Autodesk Inventor part; units mm, degrees
ref_plane "YZ Plane" through (0, 0, 0) normal (1, 0, 0) x (0, 1, 0)
ref_plane "XZ Plane" through (0, 0, 0) normal (0, 1, 0) x (-1, 0, 0)
ref_plane "XY Plane" through (0, 0, 0) normal (0, 0, 1) x (1, 0, 0)
sketch "Sketch1" plane through (0, 0, 0) normal (0, 0, 1) x (1, 0, 0)
  line L0 (232, 157.1) -> (-18, 157.1)
  line L1 (-18, 157.1) -> (-18, -92.9)
  line L2 (-18, -92.9) -> (232, -92.9)
  line L3 (232, -92.9) -> (232, 157.1)
  line L4 (-18, -42.8) -> (0, -42.8)
  line L5 (0, -42.8) -> (0, -92.9)
  line L6 (0, -92.9) -> (-18, -92.9)
  line L7 (-18, -92.9) -> (-18, -42.8)
  line L8 (0, 107) -> (0, 64.2)
  line L9 (0, 64.2) -> (-18, 64.2)
  line L10 (-18, 64.2) -> (-18, 107)
  line L11 (76.5522, 157.3937) -> (94.5522, 157.3937)
  line L12 (-18, -42.8) -> (-18, 0)
  line L13 (-18, 0) -> (0, 0)
  line L14 (0, 0) -> (0, -42.8)
  line L15 (0, -42.8) -> (-18, -42.8)
  line L16 (-18, -42.8) -> (0, -42.8)
  line L17 (0, -42.8) -> (0, 0)
  line L18 (0, 0) -> (-18, 0)
  line L19 (-18, 0) -> (-18, -42.8)
  line L20 (0, 0) -> (-18, 0)
  line L21 (-18, 0) -> (-18, 64.2)
  line L22 (-18, 64.2) -> (0, 64.2)
  line L23 (0, 64.2) -> (0, 0)
  line L24 (-18, 64.2) -> (-18, 107)
  line L25 (0, 64.2) -> (-18, 64.2)
  line L26 (-18, 64.2) -> (-18, 107)
  line L27 (76.5522, 157.3937) -> (94.5522, 157.3937)
  line L28 (0, 107) -> (0, 64.2)
  line L29 (76.5522, 157.3937) -> (94.5522, 157.3937)
  line L30 (0, 107) -> (0, 157.1)
  line L31 (0, 157.1) -> (-18, 157.1)
  line L32 (-18, 157.1) -> (-18, 107)
  line L33 (0, 64.2) -> (0, 107)
  line L34 (0, 107) -> (-18, 107)
  line L35 (232, -92.9) -> (94.5522, -92.9)
  line L36 (-18, -92.9) -> (107, -92.9)
  line L37 (107, -92.9) -> (107, 52.5886)
  line L38 (232, 157.1) -> (232, -92.9)
  line L39 (232, -42.8) -> (214, -42.8)
  line L40 (232, -92.9) -> (232, -42.8)
  line L41 (214, -42.8) -> (214, -92.9)
  line L42 (214, 107) -> (214, 64.2)
  line L43 (214, 107) -> (214, 64.2)
  line L44 (232, 64.2) -> (232, 107)
  line L45 (232, 64.2) -> (232, 107)
  line L46 (232, 64.2) -> (232, 107)
  line L47 (214, 107) -> (214, 157.1)
  line L48 (232, 157.1) -> (232, 107)
  line L49 (214, -42.8) -> (232, -42.8)
  line L50 (232, -42.8) -> (214, -42.8)
  line L51 (214, -42.8) -> (214, 0)
  line L52 (232, -42.8) -> (232, 0)
  line L53 (232, 0) -> (214, 0)
  line L54 (232, 0) -> (232, -42.8)
  line L55 (214, 0) -> (232, 0)
  line L56 (214, 0) -> (232, 0)
  line L57 (214, 64.2) -> (214, 0)
  line L58 (214, 64.2) -> (232, 64.2)
  line L59 (232, 0) -> (232, 64.2)
  line L60 (214, 64.2) -> (232, 64.2)
  line L61 (232, 64.2) -> (214, 64.2)
  line L62 (214, 0) -> (214, -42.8)
  line L63 (214, 64.2) -> (214, 107)
  line L64 (214, 107) -> (232, 107)
  line L65 (214, 157.1) -> (0, 157.1)
  line L66 (0, 157.1) -> (0, 139.1)
  line L67 (0, 139.1) -> (214, 139.1)
  line L68 (214, 139.1) -> (214, 157.1)
  line L69 (232, 157.1) -> (-18, 157.1)
  line L70 (-18, 157.1) -> (-18, 139.1)
  line L71 (-18, 139.1) -> (232, 139.1)
  line L72 (232, 139.1) -> (232, 157.1)
  line L73 (232, -92.9) -> (-18, -92.9)
  line L74 (-18, -92.9) -> (-18, -74.9)
  line L75 (-18, -74.9) -> (232, -74.9)
  line L76 (232, -74.9) -> (232, -92.9)
  point P0 (0, 0)
  point P1 (214, 0)
  point P2 (0, -74.9)
  point P3 (214, -74.9)
  dimension "d0" = 18
  dimension "d1" = 42.8
  dimension "d2" = 125
  dimension "d4" = 18
  dimension "d5" = 18
extrude "Plate1" add sketch "Sketch1" along normal blind 18 contours L47 L42 L57 L51 L41 L75 L5 L14 L23 L8 L30 L67 | L3 L58 L42 L64 | L8 L9 L1 L34 | L3 L39 L51 L53 | L14 L4 L1 L13
equation "\"d3\" = Thickness"
equation "\"BendRadius\" = Thickness"
equation "\"BendReliefWidth\" = Thickness"
equation "\"BendReliefDepth\" = 0.5 * Thickness"
equation "\"CornerReliefSize\" = 4 * Thickness"
equation "\"MinimumRemnant\" = 2 * Thickness"
equation "\"TransitionRadius\" = BendRadius"
equation "\"JacobiRadiusSize\" = BendRadius"
equation "\"GapSize\" = Thickness"
properties part number "7"
Part model, mm, in its own coordinate system. A direction names the side the tool comes from. Give positions to 0.01 mm unless a question says otherwise; leave off trailing zeros. Order: outer loops, then holes, each group sorted by start corner. A loop starts at its lowest first (then second) coordinate and runs counter-clockwise, first axis right, second up. Notation, with made-up numbers: (12, 1.5) -> (42, 1.5) arc R35 cw to (42, 36.5) -> close; hole circle Ø3 at (-27, 82.25). An arc over 180 degrees is marked (long way). Use one line per item in the form item = value.
(1) Pull direction Y, two halves, no side cores. Call faces 1 (the face through (106, -74.9, 9)), 2 (the face through (-9, 0, 9)), 3 (the face through (105, 34, 18)), 4 (the face through (223, 107, 9)): +Y half, -Y half, draft (parallel to the pull), parting line (faces both ways), or undercut.
Solution:
face_1 = -Y half
face_2 = undercut
face_3 = draft
face_4 = +Y half
(2) Saw through at B-B (y = 39.5). Write the cut outline in (x, z).
Solution:
outline = (0, 0) -> (214, 0) -> (214, 18) -> (0, 18) -> close
(3) Flat gauge pins, fed straight in: P1, Ø5, axis at y = 3.5, z = 3, coming from the -X side; P2, Ø4, axis at x = 27.5, y = 81, coming from the -Z side; P3, Ø9, axis at x = -5.5, z = 11.5, coming from the -Y side; P4, Ø5.5, axis at x = 219, z = 11, coming from the +Y side. Where does each tip first touch, or does it go through?
Solution:
P1 = 0
P2 = 0
P3 = -42.8
P4 = 107
(4) Drill centre line: line 1 (X direction, y = 42.5, z = 2.25). Where is it in solid material? Low to high. Write a range as from..to.
Solution:
line_1 = 0..214
(5) Tool access for faces 5 (the face through (214, 123, 9)), 6 (the face through (0, 123, 9)), 7 (the face through (214, -59, 9)), 8 (the face through (-9, 64.2, 9)): list every direction of +Z, -Z, +X, -X, +Y, -Y with a clear straight run to the whole face (end or side of a thin tool).
Solution:
face_5 = +Z, -Z, +X, +Y
face_6 = +Z, -Z, -X, +Y
face_7 = +Z, -Z, +X, -Y
face_8 = +Z, -Z, -X
(6) Saw through at A-A (z = 9). Write the cut outline in (x, y).
Solution:
outline = (-18, -42.8) -> (0, -42.8) -> (0, -74.9) -> (214, -74.9) -> (214, -42.8) -> (232, -42.8) -> (232, 0) -> (214, 0) -> (214, 64.2) -> (232, 64.2) -> (232, 107) -> (214, 107) -> (214, 139.1) -> (0, 139.1) -> (0, 107) -> (-18, 107) -> (-18, 64.2) -> (0, 64.2) -> (0, 0) -> (-18, 0) -> close
